CAD build for the part. Positions are in the model's coordinates, mm. Face numbers are marked on the shaded views. A direction names the side the tool comes from. Coordinates: 2 decimals unless noted, no trailing zeros. Write each loop counter-clockwise with the first axis right and the second up, starting at its lowest first coordinate (ties: lowest second). Pieces come first, ordered by that corner, then holes.
```python
from build123d import *

# Parameters (mm, degrees)
F1_DEPTH    = 48
F2_SIZE     = 6
F3_T1_DEPTH = 53
F3_T3_DEPTH = 54.5281651471
F3_T5_DEPTH = 52.4600037496


# Not quite as in the source:
# - a fillet or chamfer that OpenCascade refuses, or shapes differently, is made with other operations: its cross-section is extruded or revolved along the edge and cut away or added
# - a feature names something its author has since deleted; it is built from what else it names


with BuildPart() as f1:
    # F0 (on Top) → F1 (new body)
    with BuildSketch(Plane.XY):
        with BuildLine():
            Line((0, 4), (0, 0))
            Line((0, 0), (2, 0))
            Line((2, 0), (2, 4))
            ThreePointArc((2, 4), (3.0020118724, 5.3950578705), (4.6095750202, 6))
            ThreePointArc((4.6095750202, 6), (4.8047875101, 6.0064362795), (5, 6))
            Line((5, 6), (15, 6))
            ThreePointArc((15, 6), (18.4461762663, 3.9255722455), (19.6880345723, 0.0997168751))
            ThreePointArc((19.6880345723, 0.0997168751), (19.6856381883, 0.0498470868), (19.6828086323, 0))
            Line((19.6828086323, 0), (19.4207697359, -5))
            ThreePointArc((19.4207697359, -5), (18.9661763427, -5.5793756098), (18.26629109, -5.8084866821))
            Line((18.26629109, -5.8084866821), (16.1894012844, -5.3289988895))
            ThreePointArc((16.1894012844, -5.3289988895), (15.6261580996, -4.6575642289), (15.4106099526, -3.8080900476))
            ThreePointArc((15.4106099526, -3.8080900476), (15.4127500759, -3.6584901874), (15.4262591199, -3.5094861471))
            Line((15.4262591199, -3.5094861471), (15.4524630095, -3.0094861471))
            ThreePointArc((15.4524630095, -3.0094861471), (14.9662231771, -0.7637354985), (13.5283299865, 1.0285502831))
            Line((13.5283299865, 1.0285502831), (12.346313856, -0.5859939341))
            ThreePointArc((12.346313856, -0.5859939341), (12.5114130289, -0.7045010308), (12.6663410631, -0.8360265911))
            ThreePointArc((12.6663410631, -0.8360265911), (13.2467923067, -1.6369828382), (13.4711592073, -2.6003695984))
            ThreePointArc((13.4711592073, -2.6003695984), (13.4688331774, -2.8053678054), (13.4497183175, -3.0094861471))
            Line((13.4497183175, -3.0094861471), (13.4235144279, -3.5094861471))
            Line((13.4235144279, -3.5094861471), (13.4164237789, -3.6447837895))
            ThreePointArc((13.4164237789, -3.6447837895), (14.1205058655, -5.8682370303), (16.0652377732, -7.1556739049))
            Line((16.0652377732, -7.1556739049), (16.1894012844, -7.1843393101))
            Line((16.1894012844, -7.1843393101), (18.26629109, -7.6638271027))
            ThreePointArc((18.26629109, -7.6638271027), (20.3764129686, -6.9618705168), (21.4235144279, -5))
            Line((21.4235144279, -5), (21.6855533243, 0))
            ThreePointArc((21.6855533243, 0), (19.8249274325, 5.2386247512), (15, 8))
            Line((15, 8), (7, 8))
            Line((7, 8), (7, 14))
            Line((7, 14), (5, 14))
            Line((5, 14), (5, 8))
            Line((5, 8), (4.7983737082, 8))
            ThreePointArc((4.7983737082, 8), (1.6976247354, 6.8415893063), (0, 4))
        make_face()
    extrude(amount=F1_DEPTH)

    # F2
    f2_edges = [f1.edges().sort_by_distance(p)[0] for p in [
        (6, 14, 48),
        (6, 14, 0),
    ]]
    chamfer(f2_edges, length=F2_SIZE)

    # F3: fillet of radius 1 on 4 edges, made by hand

    # F3_s2 → F3_t1 (cut)
    with BuildSketch(Plane.XY.offset(-2.5)):
        with BuildLine():
            ThreePointArc((0, 1), (0.2928932188, 0.2928932188), (1, 0))
            Line((1, 0), (0, 0))
            Line((0, 0), (0, 1))
        make_face()
        with BuildLine():
            ThreePointArc((1, 0), (1.7071067812, 0.2928932188), (2, 1))
            Line((2, 1), (2, 0))
            Line((2, 0), (1, 0))
        make_face()
    extrude(amount=F3_T1_DEPTH, mode=Mode.SUBTRACT)

    # F3_s4 → F3_t3 (cut)
    with BuildSketch(Plane.XY.offset(-3.2640825735)):
        with BuildLine():
            ThreePointArc((12.8383454605, 0.0860838499), (13.6381253577, 0.495339622), (14.4436338584, 0.0974775525))
            ThreePointArc((14.4436338584, 0.0974775525), (14.0164512092, 0.5929671699), (13.5283299865, 1.0285502831))
            Line((13.5283299865, 1.0285502831), (12.8383454605, 0.0860838499))
        make_face()
    extrude(amount=F3_T3_DEPTH, mode=Mode.SUBTRACT)

    # F3_s6 → F3_t5 (cut)
    with BuildSketch(Plane.XY.offset(-2.2300018748)):
        with BuildLine():
            ThreePointArc((12.9064405307, -1.0905635453), (12.6804805888, -0.4840892178), (12.8732356835, 0.1337412433))
            Line((12.8732356835, 0.1337412433), (12.346313856, -0.5859939341))
            ThreePointArc((12.346313856, -0.5859939341), (12.6455057343, -0.8170439967), (12.9064405307, -1.0905635453))
        make_face()
    extrude(amount=F3_T5_DEPTH, mode=Mode.SUBTRACT)


solid = f1.part
```
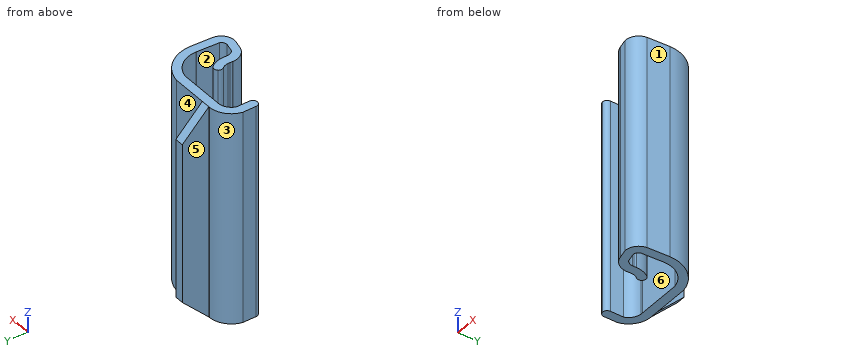
Item 1: Saw through at D-D, the plane x = 6.5. Write the cut outline in (y, z).
Item 2: Saw through at B-B, the plane x = 17.5. Write the cut outline in (y, z).
Item 3: Saw through at A-A, the plane z = 31. Write the cut outline in (x, y).
Item 4: Saw through at C-C, the plane y = -0.5. Write the cut outline in (x, z), and give its area (3 significant figures).
Item 5: Which spindle directions (+Z, -Z, +X, -X, +Y, -Y) get a long thin tool onto all of the face, cutting with end or side? Do the marked faces 4, 5 and 6. Say none if no direction does.
Item 6: Flat gauge pins, fed straight in: pin 1 Ø8 at (y, z) = (-5.5, 41) entering from -X; pin 2 Ø12 at (x, z) = (19, 16) entering from +Y; pin 3 Ø2 at (y, z) = (6, 36.5) entering from -X. Where does each tip first touch, or does it go through?
Item 7: Wall check: line 1 along X through (y, z) = (13, 14.5); line 2 along X through (y, z) = (-0.5, 35); line 3 along X through (y, z) = (-1.5, 22). Give the ranges that are in metal, low to high.
Item 8: Two-plate mould, pull along Y, no slides. Class the marked faces 1, 2 and 3: +Y half, -Y half, draft (parallel to the pull), parting line (faces both ways), or undercut.
Working result:
1. outline: (6, 0) - (8, 0) - (14, 6) - (14, 42) - (8, 48) - (6, 48) - close
2. outline: (-7.49, 0) - (-5.63, 0) - (-5.63, 48) - (-7.49, 48) - close; (4.87, 0) - (7.14, 0) - (7.14, 48) - (4.87, 48) - close
3. outline: (0, 1) arc R1 ccw to (2, 1) - (2, 4) arc R2.96 cw to (5, 6) - (15, 6) arc R5.75 cw to (19.68, 0) - (19.42, -5) arc R1.27 cw to (18.27, -5.81) - (16.19, -5.33) arc R1.97 cw to (15.43, -3.51) - (15.45, -3.01) arc R5.01 ccw to (14.44, 0.1) arc R1 ccw to (12.86, 0.11) arc R1 ccw to (12.91, -1.09) arc R2.5 cw to (13.45, -3.01) - (13.42, -3.64) arc R3.5 ccw to (16.07, -7.16) - (18.27, -7.66) arc R3 ccw to (21.42, -5) - (21.69, 0) arc R8 ccw to (15, 8) - (7, 8) - (7, 14) - (5, 14) - (5, 8) - (4.8, 8) arc R5 ccw to (0, 4) - close
4. outline: (12.68, 0) - (14.83, 0) - (14.83, 48) - (12.68, 48) - close; (19.66, 0) - (21.66, 0) - (21.66, 48) - (19.66, 48) - close
4. area: 199 mm2
5. face 4: +Z, -Z, +X, +Y
5. face 5: +Z, -Z, -X, +Y
5. face 6: +Z, -Z
6. pin 1: stops at x = 13.18
6. pin 2: stops at y = 8
6. pin 3: stops at x = 0.32
7. line 1: x = 5 to 7
7. line 2: x = 12.68 to 14.83, 19.66 to 21.66
7. line 3: x = 13.18 to 15.25, 19.6 to 21.61
8. face 1: -Y half
8. face 2: undercut
8. face 3: +Y half
